Geometry: final body of the model. Coordinates: model frame, mm. A direction names the side the tool comes from. Give positions to 0.01 mm unless a question says otherwise; leave off trailing zeros. Loops run counter-clockwise (first coordinate to the right, second up) from the corner with the lowest first, then second, coordinate; pieces in that order, holes last.
from build123d import *

# Parameters (mm, degrees)
F0_W     = 88.395819068
F0_H     = 44.2917048931
F1_DEPTH = 6.35
F2_R     = 9.5460938565
F3_DEPTH = 99.0852161
F4_R     = 4.7953323776
F5_DEPTH = 144.5512078


# Not quite as in the source:
# - an extrude ends at something that could not be found from the text; its depth is read off the source's solid


with BuildPart() as f1:
    # F0 (on Top) → F1 (new body)
    with BuildSketch(Plane.XY):
        with Locations((-1.4388076961, -22.1458524466)):
            Rectangle(F0_W, F0_H)
    extrude(amount=F1_DEPTH)

    # F2 (on face) → F3 (join, through all)
    with BuildSketch(Plane.XY.offset(6.35)):
        with Locations((0, -20.7415707409)):
            Circle(F2_R)
    extrude(amount=F3_DEPTH)

    # F4 (on face) → F5 (join, through all)
    with BuildSketch(Plane.XY.offset(105.4352161291)):
        with Locations((0, -20.7415707409)):
            Circle(F4_R)
    extrude(amount=F5_DEPTH)


solid = f1.part
Item 1: Set-up query: faces 1 (the face through (0, -21, 249.986)), 2 (the face through (-1.243, -11.277, 55.199)). Return all of +Z, -Z, +X, -X, +Y, -Y with unobstructed straight access to the full face (end or side cutting, diameter ignored); none if empty.
Values follow:
face 1: +Z, +X, -X, +Y, -Y
face 2: +Z
Item 2: Ray query, probe 1 along Z at (x, y) = (-20, -6.5); probe 2 along X at (y, z) = (-21, 134.5); probe 3 along X at (y, z) = (-20, 95.5). Return the intervals inside material, ascending.
Values follow:
probe 1: z = 0 to 6.35
probe 2: x = -4.79 to 4.79
probe 3: x = -9.52 to 9.52
Item 3: Section query A-A on x = 0. Return loops of the section in (y, z).
Values follow:
outline: (-44.29, 0) - (0, 0) - (0, 6.35) - (-11.2, 6.35) - (-11.2, 105.44) - (-15.95, 105.44) - (-15.95, 249.99) - (-25.54, 249.99) - (-25.54, 105.44) - (-30.29, 105.44) - (-30.29, 6.35) - (-44.29, 6.35) - close
Item 4: Section query C-C on z = 35.5. Return loops of the section in (x, y), plus the area to 3 significant figures.
Values follow:
outline: circle Ø19.09 at (0, -20.74)
area: 286 mm2
Item 5: Pin query (flat end, axial travel): pin 1 (12 mm diameter, centred on y = -31, z = 202.5, fed in from -X); pin 2 (8 mm diameter, centred on y = -30.5, z = 66, fed in from +X); pin 3 (10 mm diameter, centred on y = -27, z = 107, fed in from -X). Return the tip coordinate at first contact, or that it passes through.
Values follow:
pin 1: stops at x = -2.2
pin 2: stops at x = 7.61
pin 3: stops at x = -9.43
Item 6: Section query D-D on x = -15. Return loops of the section in (y, z).
Values follow:
outline: (-44.29, 0) - (0, 0) - (0, 6.35) - (-44.29, 6.35) - close
Item 7: Section query B-B on y = -6. Return loops of the section in (x, z).
Values follow:
outline: (-45.64, 0) - (42.76, 0) - (42.76, 6.35) - (-45.64, 6.35) - close
